```python
from build123d import *

# Parameters (mm, degrees)
ESQUISSE1_R        = 0.5
BOSS_EXTRU_1_DEPTH = 1.5


with BuildPart() as part:
    # Esquisse1 → Boss.-Extru.1 (new body)
    with BuildSketch(Plane.XY):
        Polygon((0, 0), (56.5, 0), (56.5, 6.7), (55.5, 6.7), (55.5, 12.3), (56.5, 12.3), (56.5, 19), (0, 19), align=None)
        with Locations((1, 18)):
            Circle(ESQUISSE1_R, mode=Mode.SUBTRACT)
        with Locations((3.54, 18)):
            Circle(ESQUISSE1_R, mode=Mode.SUBTRACT)
        with Locations((6.08, 18)):
            Circle(ESQUISSE1_R, mode=Mode.SUBTRACT)
        with Locations((8.62, 18)):
            Circle(ESQUISSE1_R, mode=Mode.SUBTRACT)
        with Locations((11.16, 18)):
            Circle(ESQUISSE1_R, mode=Mode.SUBTRACT)
        with Locations((13.7, 18)):
            Circle(ESQUISSE1_R, mode=Mode.SUBTRACT)
        with Locations((16.24, 18)):
            Circle(ESQUISSE1_R, mode=Mode.SUBTRACT)
        with Locations((18.78, 18)):
            Circle(ESQUISSE1_R, mode=Mode.SUBTRACT)
        with Locations((21.32, 18)):
            Circle(ESQUISSE1_R, mode=Mode.SUBTRACT)
        with Locations((23.86, 18)):
            Circle(ESQUISSE1_R, mode=Mode.SUBTRACT)
        with Locations((26.4, 18)):
            Circle(ESQUISSE1_R, mode=Mode.SUBTRACT)
        with Locations((28.94, 18)):
            Circle(ESQUISSE1_R, mode=Mode.SUBTRACT)
        with Locations((31.48, 18)):
            Circle(ESQUISSE1_R, mode=Mode.SUBTRACT)
        with Locations((34.02, 18)):
            Circle(ESQUISSE1_R, mode=Mode.SUBTRACT)
        with Locations((36.56, 18)):
            Circle(ESQUISSE1_R, mode=Mode.SUBTRACT)
        with Locations((39.1, 18)):
            Circle(ESQUISSE1_R, mode=Mode.SUBTRACT)
        with Locations((31.48, 15.46)):
            Circle(ESQUISSE1_R, mode=Mode.SUBTRACT)
        with Locations((28.94, 15.46)):
            Circle(ESQUISSE1_R, mode=Mode.SUBTRACT)
        with Locations((26.4, 15.46)):
            Circle(ESQUISSE1_R, mode=Mode.SUBTRACT)
        with Locations((23.86, 15.46)):
            Circle(ESQUISSE1_R, mode=Mode.SUBTRACT)
        with Locations((21.32, 15.46)):
            Circle(ESQUISSE1_R, mode=Mode.SUBTRACT)
        with Locations((18.78, 15.46)):
            Circle(ESQUISSE1_R, mode=Mode.SUBTRACT)
        with Locations((16.24, 15.46)):
            Circle(ESQUISSE1_R, mode=Mode.SUBTRACT)
        with Locations((13.7, 15.46)):
            Circle(ESQUISSE1_R, mode=Mode.SUBTRACT)
        with Locations((11.16, 15.46)):
            Circle(ESQUISSE1_R, mode=Mode.SUBTRACT)
        with Locations((31.48, 7.84)):
            Circle(ESQUISSE1_R, mode=Mode.SUBTRACT)
        with Locations((28.94, 7.84)):
            Circle(ESQUISSE1_R, mode=Mode.SUBTRACT)
        with Locations((26.4, 7.84)):
            Circle(ESQUISSE1_R, mode=Mode.SUBTRACT)
        with Locations((23.86, 7.84)):
            Circle(ESQUISSE1_R, mode=Mode.SUBTRACT)
        with Locations((21.32, 7.84)):
            Circle(ESQUISSE1_R, mode=Mode.SUBTRACT)
        with Locations((18.78, 7.84)):
            Circle(ESQUISSE1_R, mode=Mode.SUBTRACT)
        with Locations((16.24, 7.84)):
            Circle(ESQUISSE1_R, mode=Mode.SUBTRACT)
        with Locations((13.7, 7.84)):
            Circle(ESQUISSE1_R, mode=Mode.SUBTRACT)
        with Locations((11.16, 7.84)):
            Circle(ESQUISSE1_R, mode=Mode.SUBTRACT)
        with Locations((23.86, 1.49)):
            Circle(ESQUISSE1_R, mode=Mode.SUBTRACT)
        with Locations((21.32, 1.49)):
            Circle(ESQUISSE1_R, mode=Mode.SUBTRACT)
        with Locations((18.78, 1.49)):
            Circle(ESQUISSE1_R, mode=Mode.SUBTRACT)
        with Locations((16.24, 1.49)):
            Circle(ESQUISSE1_R, mode=Mode.SUBTRACT)
        with Locations((13.7, 1.49)):
            Circle(ESQUISSE1_R, mode=Mode.SUBTRACT)
        with Locations((11.16, 1.49)):
            Circle(ESQUISSE1_R, mode=Mode.SUBTRACT)
        with Locations((26.4, 1.49)):
            Circle(ESQUISSE1_R, mode=Mode.SUBTRACT)
        with Locations((36.56, 1.49)):
            Circle(ESQUISSE1_R, mode=Mode.SUBTRACT)
        with Locations((1, 1.49)):
            Circle(ESQUISSE1_R, mode=Mode.SUBTRACT)
        with Locations(Location((55.5, 1.49, 0), (0, 0, 180))):
            Circle(ESQUISSE1_R, mode=Mode.SUBTRACT)
        with Locations(Location((45.34, 1.49, 0), (0, 0, 180))):
            Circle(ESQUISSE1_R, mode=Mode.SUBTRACT)
        with Locations((3.54, 5.3)):
            Circle(ESQUISSE1_R, mode=Mode.SUBTRACT)
        with Locations((3.54, 7.84)):
            Circle(ESQUISSE1_R, mode=Mode.SUBTRACT)
        with Locations((3.54, 10.38)):
            Circle(ESQUISSE1_R, mode=Mode.SUBTRACT)
        with Locations((52.7, 9.5)):
            Circle(ESQUISSE1_R, mode=Mode.SUBTRACT)
        with Locations((47.5, 14.5)):
            Circle(ESQUISSE1_R, mode=Mode.SUBTRACT)
        with Locations((47.5, 12.3)):
            Circle(ESQUISSE1_R, mode=Mode.SUBTRACT)
        with Locations(Location((47.5, 4.5, 0), (0, 0, 180))):
            Circle(ESQUISSE1_R, mode=Mode.SUBTRACT)
        with Locations(Location((47.5, 6.7, 0), (0, 0, 180))):
            Circle(ESQUISSE1_R, mode=Mode.SUBTRACT)
        with Locations((7.985, 14.19)):
            Circle(ESQUISSE1_R, mode=Mode.SUBTRACT)
        with Locations((7.985, 9.11)):
            Circle(ESQUISSE1_R, mode=Mode.SUBTRACT)
    extrude(amount=BOSS_EXTRU_1_DEPTH)


solid = part.part
```
CAD build for the part. Positions are in the model's coordinates, mm. Round coordinates to 2 decimals unless told otherwise and drop trailing zeros. Order: outer loops, then holes, each group sorted by start corner. A loop starts at its lowest first (then second) coordinate and runs counter-clockwise, first axis right, second up. Notation, with made-up numbers: (-3.75, 38.25) -> (46.25, 38.25) arc R21 cw to (46.25, 74.25) -> close; hole circle Ø9 at (36.5, -38). An arc over 180 degrees is marked (long way). One line per question, with ' | ' between items.
Q1. Slice it at B-B (x = 52.7). Write the cut outline in (y, z).
Completed:
outline: (0, 0) -> (9, 0) -> (9, 1.5) -> (0, 1.5) -> close; (10, 0) -> (19, 0) -> (19, 1.5) -> (10, 1.5) -> close
Q2. Probe probe 1 along Y at (x, z) = (47.5, 1.15); probe 2 along Y at (x, z) = (36.56, 0.45); probe 3 along Y at (x, z) = (13.7, 0.3). List the from-to ranges inside material, lowest first.
Completed:
probe 1: y = 0 to 4, 5 to 6.2, 7.2 to 11.8, 12.8 to 14, 15 to 19 | probe 2: y = 0 to 0.99, 1.99 to 17.5, 18.5 to 19 | probe 3: y = 0 to 0.99, 1.99 to 7.34, 8.34 to 14.96, 15.96 to 17.5, 18.5 to 19
Q3. Two-plate mould, pull along X, no slides. Class faces 1 (the cylindrical face through (31.111, 18.338, 0.74)), 2 (the flat face through (28, 0, 1)): released by +X, released by -X, zero draft, split by the parting line, or undercut.
Completed:
face 1: undercut | face 2: zero draft
Q4. Slice it at A-A (x = 1). Write the cut outline in (y, z), then the cut area to 3 significant figures.
Completed:
outline: (0, 0) -> (0.99, 0) -> (0.99, 1.5) -> (0, 1.5) -> close; (1.99, 0) -> (17.5, 0) -> (17.5, 1.5) -> (1.99, 1.5) -> close; (18.5, 0) -> (19, 0) -> (19, 1.5) -> (18.5, 1.5) -> close | area: 25.5 mm^2
Q5. Slice it at C-C (z = 1.15). Give the number of separate pieces and of enclosed holes in the cut face, then the cut area to 3 significant figures.
Completed:
separate pieces: 1 | enclosed holes: 55 | area: 1,020 mm^2
